Build history of the part. All positions in model axes, mm. Face numbers are marked on the shaded views. A direction names the side the tool comes from. Give positions to 0.01 mm unless a question says otherwise; leave off trailing zeros. Loops run counter-clockwise (first coordinate to the right, second up) from the corner with the lowest first, then second, coordinate; pieces in that order, holes last. Notation, with made-up numbers: (4.5, 80.5) -> (34.5, 80.5) arc R27 cw to (34.5, 109.5) -> close; hole circle Ø10 at (53.25, 48.25). An arc over 180 degrees is marked (long way). Answer as a JSON object with one key per item and string values. Group by question number.
Q1. Band-saw the part on B-B, the plane y = -5. Write the cut outline in (x, z).
Q2. Band-saw the part on A-A, the plane z = -6.35. Write the cut outline in (x, y) (3 decimals), plus the area to 3 significant figures.
Q3. Band-saw the part on C-C, the plane z = 28. Write the cut outline in (x, y).
Q4. Tool access for the marked faces 1, 2, 3, 4 and 5: list every direction of +Z, -Z, +X, -X, +Y, -Y with a clear straight run to the whole face (end or side of a thin tool).
Q5. Band-saw the part on D-D, the plane x = 5.5. Write the cut outline in (y, z) (3 decimals), plus the area to 3 significant figures.
Q6. Wall check: probe 1 along Z at (x, y) = (17, -6); probe 2 along Z at (x, y) = (15.5, -1.5); probe 3 along Y at (x, z) = (8.5, 5). Give the ranges that are in metal, low to high. Write a range as from..to.
Q7. Two-plate mould, pull along Z, no slides. Class the marked faces 6, 7 and 8: pulls with the +Z half, pulls with the -Z half, needs draft (parallel to the pull), parting line crosses it, or undercut.
Q8. Drop flat-ended pins along their axis: pin 1 (15 mm diameter, centred on x = 9, z = 13, fed in from -Y); pin 2 (2 mm diameter, centred on x = 17.5, z = 1.5, fed in from +Y); pin 3 (3 mm diameter, centred on x = 4.5, y = 2, fed in from -Z). Give the stop position or say it passes through.
from build123d import *

# Parameters (mm, degrees)
F1_DEPTH = 6.35
F2_R     = 6.858
F3_DEPTH = 10.16
F4_R     = 6.858
F5_DEPTH = 10.16
F6_R     = 5.08
F7_DEPTH = 30.481
F8_R     = 2.54
F9_DEPTH = 25.4


with BuildPart() as f1:
    # F0 (on Front) → F1 (new body)
    with BuildSketch(Plane.XZ):
        with BuildLine():
            Line((0, 25.037667), (0, 0))
            Line((0, 0), (30.48, 0))
            Line((30.48, 0), (30.48, 25.575707))
            ThreePointArc((30.48, 25.575707), (15.016074, 37.992138), (0, 25.037667))
        make_face()
    extrude(amount=F1_DEPTH)

    # F2 (on face) → F3 (join)
    with BuildSketch(Plane.YZ.offset(30.48)):
        with Locations((-3.175, -6.35)):
            Circle(F2_R)
    extrude(amount=-F3_DEPTH)

    # F4 (on face) → F5 (join)
    with BuildSketch(Plane(origin=(0, 0, 0), x_dir=(0, -1, 0), z_dir=(-1, 0, 0))):
        with Locations((3.175, -6.35)):
            Circle(F4_R)
    extrude(amount=-F5_DEPTH)

    # F6 (on face) → F7 (cut, through all)
    with BuildSketch(Plane.YZ.offset(30.48)):
        with Locations((-3.175, -6.35)):
            Circle(F6_R)
    extrude(amount=-F7_DEPTH, mode=Mode.SUBTRACT)

    # F8 (on face) → F9 (cut)
    with BuildSketch(Plane.XZ.offset(6.35)):
        with Locations((15.016074, 29.962173)):
            Circle(F8_R)
        with Locations((15.016074, 11.774546)):
            Circle(F8_R)
    extrude(amount=-F9_DEPTH, mode=Mode.SUBTRACT)


solid = f1.part
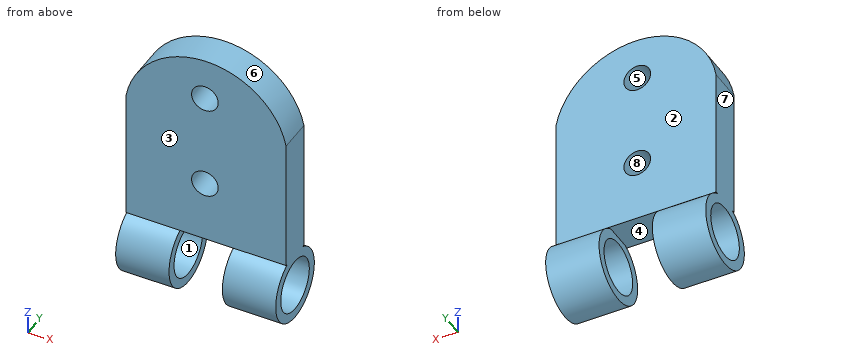
Worked answers:
{
 "1": {"outline": "(0, -12.96) -> (10.16, -12.96) -> (10.16, -11.09) -> (0, -11.09) -> close; (0, -1.61) -> (10.16, -1.61) -> (10.16, 0) -> (20.32, 0) -> (20.32, -1.61) -> (30.48, -1.61) -> (30.48, 25.58) arc R15.5 ccw to (0, 25.04) -> close; (20.32, -12.96) -> (30.48, -12.96) -> (30.48, -11.09) -> (20.32, -11.09) -> close; hole circle Ø5.08 at (15.02, 11.77); hole circle Ø5.08 at (15.02, 29.96)"},
 "2": {"outline": "(0, -10.033) -> (10.16, -10.033) -> (10.16, -8.255) -> (0, -8.255) -> close; (0, 1.905) -> (10.16, 1.905) -> (10.16, 3.683) -> (0, 3.683) -> close; (20.32, -10.033) -> (30.48, -10.033) -> (30.48, -8.255) -> (20.32, -8.255) -> close; (20.32, 1.905) -> (30.48, 1.905) -> (30.48, 3.683) -> (20.32, 3.683) -> close", "area": "72.3 mm2"},
 "3": {"outline": "(0.8, -6.35) -> (13.4, -6.35) -> (13.4, 0) -> (0.8, 0) -> close; (16.63, -6.35) -> (29.78, -6.35) -> (29.78, 0) -> (16.63, 0) -> close"},
 "4": {"face 1": "+X, -X", "face 2": "+Z, +X, -X, +Y", "face 3": "+Z, +X, -X, -Y", "face 4": "none", "face 5": "+Y, -Y"},
 "5": {"outline": "(-6.35, 0) -> (-5.765, 0) arc R6.858 ccw (long way) to (-0.585, 0) -> (0, 0) -> (0, 34.512) -> (-6.35, 34.512) -> close; hole circle Ø10.16 at (-3.175, -6.35)", "area": "284 mm2"},
 "6": {"probe 1": "0..10.19, 13.36..28.38, 31.55..37.9", "probe 2": "0..9.28, 14.27..27.47, 32.46..37.99", "probe 3": "-6.35..0"},
 "7": {"face 6": "pulls with the +Z half", "face 7": "needs draft", "face 8": "undercut"},
 "8": {"pin 1": "y = -6.35", "pin 2": "y = 0", "pin 3": "z = -12.14"}
}
